from build123d import *

# Parameters (mm, degrees)
SKETCH1_W               = 35
SKETCH1_H               = 21
BOSS_EXTRUDE1_DEPTH     = 15
SKETCH2_W               = 15
SKETCH2_H               = 5.4
CUT_EXTRUDE1_DEPTH      = 32.6
CUT_EXTRUDE2_DEPTH      = 5
FILLET1_R               = 1
CUT_EXTRUDE3_DEPTH      = 6
CUT_EXTRUDE3_DEPTH_BACK = 28.5
SKETCH4_W               = 25
SKETCH4_H               = 5.4


with BuildPart() as part:
    # Sketch1 → Boss-Extrude1 (new body)
    with BuildSketch(Plane(origin=(0, 0, 0), x_dir=(1, 0, 0), z_dir=(0, 1, 0))):
        Rectangle(SKETCH1_W, SKETCH1_H)
    extrude(amount=BOSS_EXTRUDE1_DEPTH)

    # Sketch2 → Cut-Extrude1 (cut)
    with BuildSketch(Plane.ZY.offset(17.5)):
        with Locations((-3, 2.7)):
            Rectangle(SKETCH2_W, SKETCH2_H)
    extrude(amount=-CUT_EXTRUDE1_DEPTH, mode=Mode.SUBTRACT)

    # Sketch3 → Cut-Extrude2 (cut)
    with BuildSketch(Plane(origin=(0, 15, 0), x_dir=(1, 0, 0), z_dir=(0, 1, 0))):
        Polygon((0.15, -0.925), (0.15, -8.575), (-2.5, -8.575), (-2.5, -6.325), (-17.5, -6.325), (-17.5, -3.175), (-2.5, -3.175), (-2.5, -0.925), align=None)
        Polygon((1.425, 10.5), (4.575, 10.5), (4.575, 5.5), (6.825, 5.5), (6.825, 2.85), (-0.825, 2.85), (-0.825, 5.5), (1.425, 5.5), align=None)
    extrude(amount=-CUT_EXTRUDE2_DEPTH, mode=Mode.SUBTRACT)

    # Fillet1
    fillet1_edges = [part.edges().sort_by_distance(p)[0] for p in [
        (-2.5, 12.5, 6.325),
        (-17.5, 12.5, 6.325),
        (-17.5, 12.5, 3.175),
        (-2.5, 12.5, 3.175),
        (-1.175, 15, 0.925),
        (-2.5, 15, 2.05),
        (-10, 15, 3.175),
        (-10, 15, 6.325),
        (-2.5, 15, 7.45),
        (-1.175, 15, 8.575),
        (0.15, 15, 4.75),
        (1.425, 12.5, -5.5),
        (4.575, 12.5, -5.5),
        (1.425, 15, -8),
        (0.3, 15, -5.5),
        (-0.825, 15, -4.175),
        (3, 15, -2.85),
        (6.825, 15, -4.175),
        (5.7, 15, -5.5),
        (4.575, 15, -8),
    ]]
    fillet(fillet1_edges, radius=FILLET1_R)

    # Sketch4 → Cut-Extrude3 (cut, two sides: drawn at the far end of the back side and taken through both)
    with BuildSketch(Plane(origin=(0, 0, 4.5), x_dir=(-1, 0, 0), z_dir=(0, 0, -1)).offset(-CUT_EXTRUDE3_DEPTH_BACK)):
        with Locations((-5, 2.7)):
            Rectangle(SKETCH4_W, SKETCH4_H)
    extrude(amount=CUT_EXTRUDE3_DEPTH + CUT_EXTRUDE3_DEPTH_BACK, mode=Mode.SUBTRACT)


solid = part.part
Work out the finished part from the listing and answer in its coordinate system (mm). A direction names the side the tool comes from. Coordinates: 2 decimals unless noted, no trailing zeros. Write each loop counter-clockwise with the first axis right and the second up, starting at its lowest first coordinate (ties: lowest second). Pieces come first, ordered by that corner, then holes. Notation, with made-up numbers: M 7,41.25 L 35,41.25 A20 cw 35,52.25 Z; hole C 25,17.5 d7. An arc over 180 degrees is marked long. Write item = value, one per line.
1. For faces 4 (the face through (-10, 12, 3.175)), 5 (the face through (-7.5, 3, 8)), 6 (the face through (-0.4, 14.8, -5.9)), determine the directions among +Z, -Z, +X, -X, +Y, -Y from which every point of the face is accessible in a straight line to the end or side of a thin tool.
Solution:
face_4 = -X, +Y
face_5 = +Z, -Z, +X, -Y
face_6 = +Y
2. Determine the mould class of faces 1 (the face through (4.876, 14.715, -8.472)), 2 (the face through (16, 3, -1.5)), 3 (the face through (-2.8, 11.97, 2.89)) for opening direction Z: released by +Z, released by -Z, zero draft, split by the parting line, or undercut.
Solution:
face_1 = zero draft
face_2 = released by +Z
face_3 = undercut
3. The part is cut by section B-B (z = -7). Determine the outline of the cut face in (x, y) (3 decimals), then the cut area to 3 significant figures.
Solution:
outline = M -17.5,5.4 L 15.1,5.4 L 15.1,0 L 17.5,0 L 17.5,15 L 5.575,15 A1 ccw 4.575,14 L 4.575,10 L 1.425,10 L 1.425,14 A1 ccw 0.425,15 L -17.5,15 Z
area = 333 mm2
4. The part is cut by section C-C (x = -13.5). Determine the outline of the cut face in (y, z) (3 decimals), then the cut area to 3 significant figures.
Solution:
outline = M 0,4.5 L 5.4,4.5 L 5.4,-10.5 L 15,-10.5 L 15,2.175 A1 ccw 14,3.175 L 10,3.175 L 10,6.325 L 14,6.325 A1 ccw 15,7.325 L 15,10.5 L 0,10.5 Z
area = 218 mm2
5. The part is cut by section A-A (y = 3). Determine the outline of the cut face in (x, z).
Solution:
outline = M -17.5,4.5 L -7.5,4.5 L -7.5,10.5 L -17.5,10.5 Z; M 15.1,-10.5 L 17.5,-10.5 L 17.5,-1.5 L 15.1,-1.5 Z
6. The part is cut by section D-D (y = 12.5). Determine the outline of the cut face in (x, z) (3 decimals).
Solution:
outline = M -17.5,-10.5 L 1.425,-10.5 L 1.425,-6.5 A1 ccw 0.425,-5.5 L -0.825,-5.5 L -0.825,-2.85 L 6.825,-2.85 L 6.825,-5.5 L 5.575,-5.5 A1 ccw 4.575,-6.5 L 4.575,-10.5 L 17.5,-10.5 L 17.5,10.5 L -17.5,10.5 L -17.5,7.325 A1 ccw -16.5,6.325 L -3.5,6.325 A1 ccw -2.5,7.325 L -2.5,8.575 L 0.15,8.575 L 0.15,0.925 L -2.5,0.925 L -2.5,2.175 A1 ccw -3.5,3.175 L -16.5,3.175 A1 ccw -17.5,2.175 Z
7. Straight lines are drawn through the part: line 1 (X direction, y = 10.5, z = -3.75) (3 decimals); line 2 (Y direction, x = 0.5, z = -3.75); line 3 (Z direction, x = 15.5, y = 4.5). For each, find the intervals that lie inside material, in ascending order. Write a range as from..to.
Solution:
line_1 = -17.5..-0.825, 6.825..17.5
line_2 = 5.4..10
line_3 = -10.5..-1.5
8. Flat-ended cylindrical pins translate along their axes: pin 1 (8.5 mm diameter, centred on x = -8.5, z = 5, fed in from +Y); pin 2 (2 mm diameter, centred on y = 11.5, z = 6, fed in from -X); pin 3 (12 mm diameter, centred on x = -4.5, z = -7, fed in from -Y); pin 4 (2.5 mm diameter, centred on x = 17, y = 2.5, fed in from +Z). Find the tip coordinate at first contact, or state that the pin passes through.
Solution:
pin_1 = 15
pin_2 = -17.45
pin_3 = 5.4
pin_4 = -1.5
